```python
from build123d import *

# Parameters (mm, degrees)
SKETCH3_W                                  = 279.4
SKETCH3_H                                  = 101.6
RECTANGLE_CUT_DEPTH                        = 5.08
SKETCH4_R                                  = 10.16
CUT_EXTRUDE2_DEPTH                         = 7.62
MIRROR3_COPY_1_SKETCH_R                    = 10.16
MIRROR3_COPY_1_DEPTH                       = 7.62
SKETCH6_W                                  = 36.068
SKETCH6_H                                  = 17.526
CUT_EXTRUDE3_DEPTH                         = 7.62
SKETCH9_W                                  = 329.627948334
SKETCH9_H                                  = 121.564544856
CUT_EXTRUDE5_DEPTH                         = 2.54
SKETCH11_R                                 = 1.4224
CUT_EXTRUDE6_DEPTH                         = 2.54
MIRROR4_AT_THE_SECOND_PLANE_COPY_1_SKETC_R = 1.4224
MIRROR4_AT_THE_SECOND_PLANE_COPY_1_DEPTH   = 2.54
SKETCH12_R                                 = 1.4224
CUT_EXTRUDE7_DEPTH                         = 2.54
SKETCH13_R                                 = 1.4224
CUT_EXTRUDE8_DEPTH                         = 2.54


with BuildPart() as part:
    # Sketch3 → Rectangle cut (new body)
    with BuildSketch(Plane(origin=(0, 0, 0), x_dir=(1, 0, 0), z_dir=(0, 1, 0))):
        Rectangle(SKETCH3_W, SKETCH3_H)
    extrude(amount=-RECTANGLE_CUT_DEPTH)

    # Sketch4 → Cut-Extrude2 (cut)
    with BuildSketch(Plane(origin=(0, 0, 0), x_dir=(1, 0, 0), z_dir=(0, 1, 0))):
        with Locations((-139.7, -50.8)):
            Circle(SKETCH4_R)
    cut_extrude2 = extrude(amount=-CUT_EXTRUDE2_DEPTH, mode=Mode.SUBTRACT)

    # mountingCorners: Cut-Extrude2 across plane
    add(cut_extrude2.mirror(Plane(origin=(0, 0, 0), x_dir=(0, 0, 1), z_dir=(1, 0, 0))), mode=Mode.SUBTRACT)

    # Mirror3: Cut-Extrude2 across plane
    add(cut_extrude2.mirror(Plane.XY), mode=Mode.SUBTRACT)

    # Mirror3 copy 1 sketch → Mirror3 copy 1 (cut)
    with BuildSketch(Plane(origin=(0, 0, 0), x_dir=(-1, 0, 0), z_dir=(0, 1, 0))):
        with Locations((-139.7, -50.8)):
            Circle(MIRROR3_COPY_1_SKETCH_R)
    extrude(amount=-MIRROR3_COPY_1_DEPTH, mode=Mode.SUBTRACT)

    # Sketch6 → Cut-Extrude3 (cut)
    with BuildSketch(Plane(origin=(0, 0, 0), x_dir=(1, 0, 0), z_dir=(0, 1, 0))):
        with Locations((-41.656, 8.001)):
            Rectangle(SKETCH6_W, SKETCH6_H)
    extrude(amount=-CUT_EXTRUDE3_DEPTH, mode=Mode.SUBTRACT)

    # Sketch9 → Cut-Extrude5 (cut)
    with BuildSketch(Plane.XZ.offset(5.08)):
        Rectangle(SKETCH9_W, SKETCH9_H)
    extrude(amount=-CUT_EXTRUDE5_DEPTH, mode=Mode.SUBTRACT)

    # Sketch11 → Cut-Extrude6 (cut)
    with BuildSketch(Plane.XZ.offset(2.54)):
        with Locations((-114.3, -45.72)):
            Circle(SKETCH11_R)
    cut_extrude6 = extrude(amount=-CUT_EXTRUDE6_DEPTH, mode=Mode.SUBTRACT)

    # Mirror4: Cut-Extrude6 across plane
    add(cut_extrude6.mirror(Plane.XY), mode=Mode.SUBTRACT)

    # Mirror4 at the second plane: Cut-Extrude6 across plane
    add(cut_extrude6.mirror(Plane(origin=(0, 0, 0), x_dir=(0, 0, 1), z_dir=(1, 0, 0))), mode=Mode.SUBTRACT)

    # Mirror4 at the second plane copy 1 sketc → Mirror4 at the second plane copy 1 (cut)
    with BuildSketch(Plane(origin=(0, -2.54, 0), x_dir=(-1, 0, 0), z_dir=(0, -1, 0))):
        with Locations((-114.3, -45.72)):
            Circle(MIRROR4_AT_THE_SECOND_PLANE_COPY_1_SKETC_R)
    extrude(amount=-MIRROR4_AT_THE_SECOND_PLANE_COPY_1_DEPTH, mode=Mode.SUBTRACT)

    # Sketch12 → Cut-Extrude7 (cut)
    with BuildSketch(Plane.XZ.offset(2.54)):
        with Locations((-134.62, 0)):
            Circle(SKETCH12_R)
    cut_extrude7 = extrude(amount=-CUT_EXTRUDE7_DEPTH, mode=Mode.SUBTRACT)

    # Mirror5: Cut-Extrude7 across plane
    add(cut_extrude7.mirror(Plane(origin=(0, 0, 0), x_dir=(0, 0, 1), z_dir=(1, 0, 0))), mode=Mode.SUBTRACT)

    # Sketch13 → Cut-Extrude8 (cut)
    with BuildSketch(Plane.XZ.offset(2.54)):
        with Locations((0, -45.72)):
            Circle(SKETCH13_R)
    cut_extrude8 = extrude(amount=-CUT_EXTRUDE8_DEPTH, mode=Mode.SUBTRACT)

    # Mirror6: Cut-Extrude8 across plane
    add(cut_extrude8.mirror(Plane.XY), mode=Mode.SUBTRACT)


solid = part.part
```
Read the model definition and answer for the solid it produces. Units are mm, in the model's axes. Give positions to 0.01 mm unless a question says otherwise; leave off trailing zeros. Write each loop counter-clockwise with the first axis right and the second up, starting at its lowest first coordinate (ties: lowest second). Pieces come first, ordered by that corner, then holes. Notation, with made-up numbers: M 83,-10 L 137,-10 A36 ccw 137,29 Z; hole C 65,6.5 d2. An arc over 180 degrees is marked long. Put each result on its own line as item: value. Start each with the question number.
1. The part is cut by section A-A, the plane x = -33. Give the vertices of the cut face in (y, z).
2. Consider line 1 along Z through (x, y) = (114.3, -1.7); line 2 along X through (y, z) = (-1.65, 45.72); line 3 along X through (y, z) = (-0.85, -4.5). Determine where each line is inside the solid, lowest interval first.
3. The part is cut by section B-B, the plane y = -1.3. Give the number of separate pieces and of enclosed holes in the cut face, and give its area (3 significant figures).
Final values:
1. outline: M -2.54,-50.8 L 0,-50.8 L 0,-16.76 L -2.54,-16.76 Z; M -2.54,0.76 L 0,0.76 L 0,50.8 L -2.54,50.8 Z
2. line 1: z = -50.8 to -47.14, -44.3 to 44.3, 47.14 to 50.8
2. line 2: x = -130.9 to -115.72, -112.88 to -1.42, 1.42 to 112.88, 115.72 to 130.9
2. line 3: x = -139.7 to -59.69, -23.62 to 139.7
3. separate pieces: 1
3. enclosed holes: 9
3. area: 27,400 mm²
